```python
from build123d import *

# Parameters (mm, degrees)
F0_W     = 304.8
F0_H     = 25.4
F1_DEPTH = 25.4
F2_W     = 22.225
F2_H     = 22.225
F3_DEPTH = 304.8
F4_R     = 2.5527
F5_DEPTH = 25.4
F6_R     = 2.5527
F7_DEPTH = 25.4


with BuildPart() as f1:
    # F0 (on Right) → F1 (new body)
    with BuildSketch(Plane.YZ):
        with Locations((78.871952, 17.516105)):
            Rectangle(F0_W, F0_H)
    extrude(amount=F1_DEPTH)

    # F2 (on face) → F3 (cut)
    with BuildSketch(Plane.XZ.offset(73.528048)):
        with Locations((12.586378, 17.516105)):
            Rectangle(F2_W, F2_H)
    extrude(amount=-F3_DEPTH, mode=Mode.SUBTRACT)

    # F4 (on face) → F5 (cut)
    with BuildSketch(Plane.XY.offset(30.216105)):
        with Locations((12.7, -60.828048)):
            Circle(F4_R)
        with Locations((12.7, -35.428048)):
            Circle(F4_R)
        with Locations((12.7, -10.028048)):
            Circle(F4_R)
        with Locations((12.7, 15.371952)):
            Circle(F4_R)
        with Locations((12.7, 40.771952)):
            Circle(F4_R)
        with Locations((12.7, 66.171952)):
            Circle(F4_R)
        with Locations((12.7, 91.571952)):
            Circle(F4_R)
        with Locations((12.7, 116.971952)):
            Circle(F4_R)
        with Locations((12.7, 142.371952)):
            Circle(F4_R)
        with Locations((12.7, 167.771952)):
            Circle(F4_R)
        with Locations((12.7, 193.171952)):
            Circle(F4_R)
        with Locations((12.7, 218.571952)):
            Circle(F4_R)
    extrude(amount=-F5_DEPTH, mode=Mode.SUBTRACT)

    # F6 (on face) → F7 (cut)
    with BuildSketch(Plane(origin=(0, 0, 0), x_dir=(0, -1, 0), z_dir=(-1, 0, 0))):
        with Locations((60.584806, 17.516105)):
            Circle(F6_R)
        with Locations((35.184806, 17.516105)):
            Circle(F6_R)
        with Locations((9.784806, 17.516105)):
            Circle(F6_R)
        with Locations((-15.615194, 17.516105)):
            Circle(F6_R)
        with Locations((-41.015194, 17.516105)):
            Circle(F6_R)
        with Locations((-66.415194, 17.516105)):
            Circle(F6_R)
        with Locations((-91.815194, 17.516105)):
            Circle(F6_R)
        with Locations((-117.215194, 17.516105)):
            Circle(F6_R)
        with Locations((-142.615194, 17.516105)):
            Circle(F6_R)
        with Locations((-168.015194, 17.516105)):
            Circle(F6_R)
        with Locations((-193.415194, 17.516105)):
            Circle(F6_R)
        with Locations((-218.815194, 17.516105)):
            Circle(F6_R)
    extrude(amount=-F7_DEPTH, mode=Mode.SUBTRACT)


solid = f1.part
```
Source: CAD feature listing. Evaluate the final solid. Frame: model axes, mm. A direction names the side the tool comes from. Give positions to 0.01 mm unless a question says otherwise; leave off trailing zeros. Loops run counter-clockwise (first coordinate to the right, second up) from the corner with the lowest first, then second, coordinate; pieces in that order, holes last. Notation, with made-up numbers: (68, -10.75) - (107, -10.75) arc R31 cw to (107, 24.25) - close; hole circle Ø2 at (87.25, 41.25). An arc over 180 degrees is marked (long way). Use CSV: the item, a comma, the result in double quotes. Start each with the question number.
1. Ray query, L1, parallel to Z at x = 3.75, y = 44; L2, parallel to X at y = 33, z = 25. Return the intervals inside material, ascending.
2. Section A-A (y = 4.5). Output: boundary loops of the cut face in (x, z), then the cut area to 3 significant figures.
3. Draft query along Z for faces 3 (the cylindrical face through (12.15, 216.08, 29.43)), 4 (the cylindrical face through (0.73, 38.58, 18.28)), 5 (the flat face through (13, 77, 30.216)). Return one class per face: +Z half, -Z half, draft (parallel to the pull), parting line (faces both ways), or undercut.
4. Reachability of faces 1 (the cylindrical face through (0.73, 89.38, 18.28)), 2 (the flat face through (12, 77, 28.629)) from +Z, -Z, +X, -X, +Y, -Y: full face, straight path, thin tool, end or side. Return the list, or none.
5. Pin query (flat end, axial travel): pin 1 (2 mm diameter, centred on y = -39.5, z = 20, fed in from -X); pin 2 (3 mm diameter, centred on x = 12.7, y = 142.37, fed in from -Z). Return the tip coordinate at first contact, or that it passes through.
6. Section B-B (x = 12.7). Count the separate pieces of the cut face and the enclosed holes in it, then the cut area to 3 significant figures.
Response:
1,L1,"4.82 to 6.4, 28.63 to 30.22"
1,L2,"0 to 1.47, 23.7 to 25.4"
2,outline,"(0, 4.82) - (25.4, 4.82) - (25.4, 30.22) - (0, 30.22) - close; hole (1.47, 6.4) - (23.7, 6.4) - (23.7, 28.63) - (1.47, 28.63) - close"
2,area,"151 mm²"
3,face 3,"draft"
3,face 4,"undercut"
3,face 5,"+Z half"
4,face 1,"+X, -X"
4,face 2,"+Y, -Y"
5,pin 1,"x = 0"
5,pin 2,"through"
6,separate pieces,"26"
6,enclosed holes,"0"
6,area,"773 mm²"
